Geometry check sheet. Reference: the model listing, model coordinates, mm. Coordinates: 2 decimals unless noted, no trailing zeros. Write each loop counter-clockwise with the first axis right and the second up, starting at its lowest first coordinate (ties: lowest second). Pieces come first, ordered by that corner, then holes.
from build123d import *

# Parameters (mm, degrees)
SKETCH1_W                   = 203.2
SKETCH1_H                   = 101.6
BOSS_EXTRUDE1_DEPTH         = 5.08
TAP_DRILL_FOR_M5X0_8_TAP1_D = 4.2


with BuildPart() as part:
    # Sketch1 → Boss-Extrude1 (new body)
    with BuildSketch(Plane(origin=(0, 0, 0), x_dir=(1, 0, 0), z_dir=(0, 1, 0))):
        with Locations((101.6, -50.8)):
            Rectangle(SKETCH1_W, SKETCH1_H)
    extrude(amount=BOSS_EXTRUDE1_DEPTH)

    # Tap Drill for M5x0.8 Tap1 (through all)
    with Locations(Plane(origin=(0, 0, 0), x_dir=(-1, 0, 0), z_dir=(0, -1, 0))):
        with Locations((-196.2, -5), (-182.2, -5), (-196.2, -25), (-182.2, -25), (-21, -5), (-7, -5), (-21, -25), (-7, -25), (-7, -76.6), (-196.2, -76.6), (-182.2, -76.6), (-182.2, -96.6), (-196.2, -96.6), (-21, -76.6), (-21, -96.6), (-7, -96.6)):
            Hole(TAP_DRILL_FOR_M5X0_8_TAP1_D / 2)


solid = part.part
1. Draft check along X on faces 1 (the cylindrical face through (23.003, 2.576, 24.369)), 2 (the flat face through (0, 3, 52)), 3 (the flat face through (100, 3, 101.6)), 4 (the cylindrical face through (181.74, 2.58, 98.65)). Enter one of: released by +X, released by -X, zero draft, split by the parting line, or undercut.
Computed values:
face 1: undercut
face 2: released by -X
face 3: zero draft
face 4: undercut
2. Sectioned sample at B-B, the plane z = 5. Record the boundary of the cut face in (x, y), and give its area (3 significant figures).
Computed values:
outline: (0, 0) - (4.9, 0) - (4.9, 5.08) - (0, 5.08) - close; (9.1, 0) - (18.9, 0) - (18.9, 5.08) - (9.1, 5.08) - close; (23.1, 0) - (180.1, 0) - (180.1, 5.08) - (23.1, 5.08) - close; (184.3, 0) - (194.1, 0) - (194.1, 5.08) - (184.3, 5.08) - close; (198.3, 0) - (203.2, 0) - (203.2, 5.08) - (198.3, 5.08) - close
area: 947 mm2
3. Gauge pin test, flat end, axial feed: pin 1 Ø2.5 at (x, z) = (182.2, 96.6) entering from +Y. Record the tip position at first contact, or that the pin passes through.
Computed values:
pin 1: passes through
4. Sectioned sample at A-A, the plane x = 196.2. Record the boundary of the cut face in (y, z).
Computed values:
outline: (0, 0) - (5.08, 0) - (5.08, 2.9) - (0, 2.9) - close; (0, 7.1) - (5.08, 7.1) - (5.08, 22.9) - (0, 22.9) - close; (0, 27.1) - (5.08, 27.1) - (5.08, 74.5) - (0, 74.5) - close; (0, 78.7) - (5.08, 78.7) - (5.08, 94.5) - (0, 94.5) - close; (0, 98.7) - (5.08, 98.7) - (5.08, 101.6) - (0, 101.6) - close
5. Thickness scan on line 1 along Z through (x, y) = (7, 1.9); line 2 along X through (y, z) = (1.4, 76.6); line 3 along X through (y, z) = (2.8, 6.5). Record the ranges inside material, lowest first.
Computed values:
line 1: z = 0 to 2.9, 7.1 to 22.9, 27.1 to 74.5, 78.7 to 94.5, 98.7 to 101.6
line 2: x = 0 to 4.9, 9.1 to 18.9, 23.1 to 180.1, 184.3 to 194.1, 198.3 to 203.2
line 3: x = 0 to 5.53, 8.47 to 19.53, 22.47 to 180.73, 183.67 to 194.73, 197.67 to 203.2
